```python
from build123d import *

# Parameters (mm, degrees)
F0_R     = 25.4
F1_DEPTH = 10.16
F2_R     = 45.72
F2_R_2   = 25.4
F3_DEPTH = 13.97
F4_R     = 5.08


with BuildPart() as f1:
    # F0 (on Front) → F1 (new body, symmetric)
    with BuildSketch(Plane.XZ):
        Circle(F0_R)
    extrude(amount=F1_DEPTH, both=True)

    # F2 (on Front) → F3 (join, symmetric)
    with BuildSketch(Plane.XZ):
        Circle(F2_R)
        Circle(F2_R_2, mode=Mode.SUBTRACT)
    extrude(amount=F3_DEPTH, both=True)

    # F4
    f4_edges = [f1.edges().sort_by_distance(p)[0] for p in [
        (-45.72, 13.97, 0),
        (-45.72, -13.97, 0),
    ]]
    fillet(f4_edges, radius=F4_R)


solid = f1.part
```
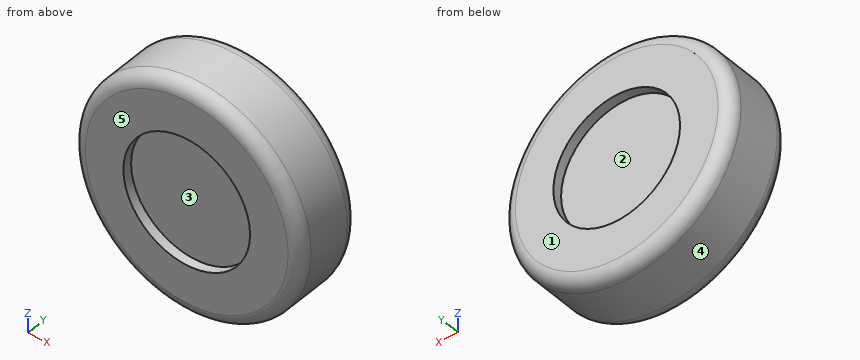
Can you work these out from the model? Positions are in its coordinate system, mm. Face numbers are marked on the shaded views. A direction names the side the tool comes from. Coordinates: 2 decimals unless noted, no trailing zeros. Loops run counter-clockwise (first coordinate to the right, second up) from the corner with the lowest first, then second, coordinate; pieces in that order, holes last. Notation, with made-up numbers: (-0.75, -3) - (32.25, -3) arc R12 ccw to (32.25, 20) - close; hole circle Ø5 at (15, 6). An arc over 180 degrees is marked (long way). Answer as CSV lines item,"result". Start each with the question number.
1) Suppose I cut it at B-B (z = 0). Please give me the cut outline in (x, y).
2) Which directions (+Z, -Z, +X, -X, +Y, -Y) give clear straight access to the entire face, cutting with the end or side of a thin tool? Please do the marked faces 1 and 2.
3) For pin 1 (1.5 mm diameter, centred on x = 15.5, y = -3.5, fed in from +Z); pin 2 (1.5 mm diameter, centred on y = 2, z = 30, fed in from +X); pin 3 (12 mm diameter, centred on y = -7.5, z = 34, fed in from +X); pin 4 (10 mm diameter, centred on x = 2, z = 24.5, fed in from +Y), each with a flat end and sliding along its axis, tell me the tip position at first contact or that it passes through.
4) Thinking about a two-plate mould opening in X: for the marked faces 3, 4 and 5, which applies, pulls with the +X half, pulls with the -X half, needs draft (parallel to the pull), parting line crosses it, or undercut?
5) Suppose I cut it at A-A (x = 0). Please give me the cut outline in (y, z).
6) I need wall thicknesses on line 1 (Z direction, x = -11.5, y = 12); line 2 (Z direction, x = 0, y = 12.55); line 3 (Y direction, x = 23.5, z = 7). Which ranges of each line are inside material? Lowest first, please. Write a range as from..to.
7) Suppose I cut it at C-C (y = -2.75). Please give me the cut outline in (x, z), plus the area to 3 significant figures.
Check result:
1,outline,"(-45.72, -8.89) arc R5.08 ccw to (-40.64, -13.97) - (-25.4, -13.97) - (-25.4, -10.16) - (25.4, -10.16) - (25.4, -13.97) - (40.64, -13.97) arc R5.08 ccw to (45.72, -8.89) - (45.72, 8.89) arc R5.08 ccw to (40.64, 13.97) - (25.4, 13.97) - (25.4, 10.16) - (-25.4, 10.16) - (-25.4, 13.97) - (-40.64, 13.97) arc R5.08 ccw to (-45.72, 8.89) - close"
2,face 1,"+Z, -Z, +X, -X, +Y"
2,face 2,"+Y"
3,pin 1,"stops at z = 43.28"
3,pin 2,"stops at x = 35.14"
3,pin 3,"stops at x = 36.14"
3,pin 4,"stops at y = 13.97"
4,face 3,"undercut"
4,face 4,"parting line crosses it"
4,face 5,"needs draft"
5,outline,"(-13.97, -40.64) arc R5.08 ccw to (-8.89, -45.72) - (8.89, -45.72) arc R5.08 ccw to (13.97, -40.64) - (13.97, -25.4) - (10.16, -25.4) - (10.16, 25.4) - (13.97, 25.4) - (13.97, 40.64) arc R5.08 ccw to (8.89, 45.72) - (-8.89, 45.72) arc R5.08 ccw to (-13.97, 40.64) - (-13.97, 25.4) - (-10.16, 25.4) - (-10.16, -25.4) - (-13.97, -25.4) - close"
6,line 1,"z = -43.15..-22.65, 22.65..43.15"
6,line 2,"z = -44.16..-25.4, 25.4..44.16"
6,line 3,"y = -10.16..10.16"
7,outline,"circle Ø91.44 at (0, 0)"
7,area,"6,570 mm²"
